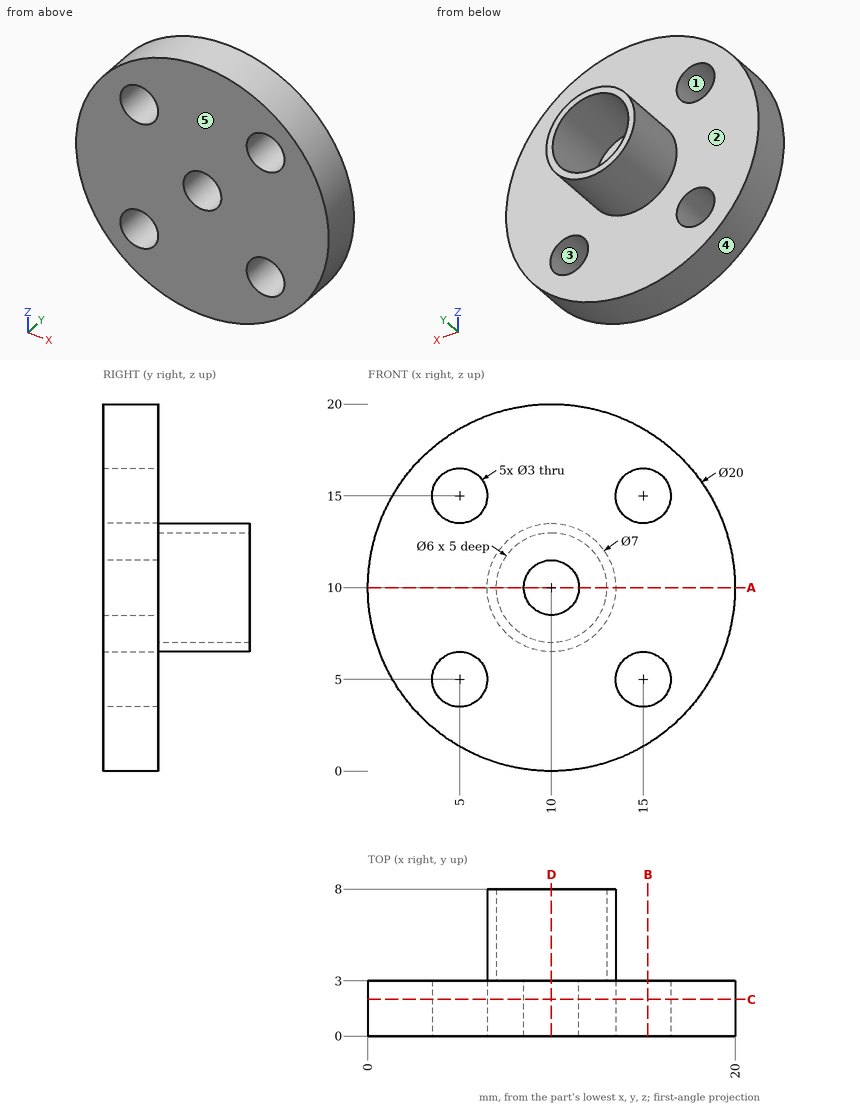
Input: dimensioned drawing with shaded views. Units: mm. Origin: part minimum x, y, z. A direction names the side the tool comes from. Coordinates: 2 decimals unless noted, no trailing zeros. Write each loop counter-clockwise with the first axis right and the second up, starting at its lowest first coordinate (ties: lowest second). Pieces come first, ordered by that corner, then holes. Notation, with made-up numbers: (78, -28) -> (135, -28) arc R25 cw to (135, -1) -> close; hole circle Ø9 at (51.5, 51). An arc over 180 degrees is marked (long way). Return JSON: item names as keys, results as strings. Group by question number.
1) Ray query, line 1 along X through (y, z) = (1.9, 10); line 2 along X through (y, z) = (2.1, 5); line 3 along X through (y, z) = (5.5, 10). Return the intervals inside material, ascending.
2) Mould query, pull axis Z, two halves, no side actions, for the marked faces 3, 4 and 5. Classes: +Z half, -Z half, draft (parallel to the pull), parting line (faces both ways), or undercut.
3) Set-up query: the marked faces 1 and 2. Return all of +Z, -Z, +X, -X, +Y, -Y with unobstructed straight access to the full face (end or side cutting, diameter ignored); none if empty.
4) Section query B-B, the plane x = 15.25. Return loops of the section in (y, z), plus the area to 3 significant figures.
5) Contact query for flat-ended pins moving along their axis: P1, Ø6.5, axis at x = 10.5, z = 9.5, coming from the +Y side; P2, Ø1, axis at x = 16.5, z = 16.5, coming from the +Y side; P3, Ø2, axis at x = 16, y = 7, coming from the -Z side. Output: stop coordinate, or through.
6) Section query D-D, the plane x = 10. Return loops of the section in (y, z), plus the area to 3 significant figures.
7) Section query C-C, the plane y = 2. Return loops of the section in (x, z).
8) Section query A-A, the plane z = 10. Return loops of the section in (x, y), plus the area to 3 significant figures.
From the geometry:
{
 "1": {"line 1": "0 to 8.5, 11.5 to 20", "line 2": "1.34 to 3.5, 6.5 to 13.5, 16.5 to 18.66", "line 3": "6.5 to 7, 13 to 13.5"},
 "2": {"face 3": "undercut", "face 4": "parting line", "face 5": "draft"},
 "3": {"face 1": "+Y, -Y", "face 2": "+Y"},
 "4": {"outline": "(0, 1.49) -> (3, 1.49) -> (3, 3.52) -> (0, 3.52) -> close; (0, 6.48) -> (3, 6.48) -> (3, 13.52) -> (0, 13.52) -> close; (0, 16.48) -> (3, 16.48) -> (3, 18.51) -> (0, 18.51) -> close", "area": "33.3 mm²"},
 "5": {"P1": "y = 8", "P2": "y = 3", "P3": "through"},
 "6": {"outline": "(0, 0) -> (3, 0) -> (3, 6.5) -> (8, 6.5) -> (8, 7) -> (3, 7) -> (3, 8.5) -> (0, 8.5) -> close; (0, 11.5) -> (3, 11.5) -> (3, 13) -> (8, 13) -> (8, 13.5) -> (3, 13.5) -> (3, 20) -> (0, 20) -> close", "area": "56.0 mm²"},
 "7": {"outline": "circle Ø20 at (10, 10); hole circle Ø3 at (5, 5); hole circle Ø3 at (5, 15); hole circle Ø3 at (10, 10); hole circle Ø3 at (15, 5); hole circle Ø3 at (15, 15)"},
 "8": {"outline": "(0, 0) -> (8.5, 0) -> (8.5, 3) -> (7, 3) -> (7, 8) -> (6.5, 8) -> (6.5, 3) -> (0, 3) -> close; (11.5, 0) -> (20, 0) -> (20, 3) -> (13.5, 3) -> (13.5, 8) -> (13, 8) -> (13, 3) -> (11.5, 3) -> close", "area": "56.0 mm²"}
}
